The model under review builds one solid part; all positions refer to its coordinate system, in mm. A direction names the side the tool comes from. Round coordinates to 2 decimals unless told otherwise and drop trailing zeros. Loops run counter-clockwise (first coordinate to the right, second up) from the corner with the lowest first, then second, coordinate; pieces in that order, holes last. Notation, with made-up numbers: M 63.5,83 L 114.5,83 A22 ccw 114.5,106 Z; hole C -3,-22.75 d2. An arc over 180 degrees is marked long. Use a Markdown table: item, result. Add a question column.
```python
from build123d import *

# Parameters (mm, degrees)
SALIENTE_EXTRUIR1_DEPTH  = 22
CROQUIS3_R               = 2.5
CROQUIS3_R_2             = 4.5
CORTAR_EXTRUIR2_DEPTH    = 1.5
CROQUIS4_R               = 2.5
CORTAR_EXTRUIR3_DEPTH    = 18
CROQUIS5_R               = 4.05861195
CORTAR_EXTRUIR4_DEPTH    = 1.5
CROQUIS6_R               = 2.5
CORTAR_EXTRUIR5_DEPTH    = 15
SALIENTE_EXTRUIR2_DEPTH  = 19
CROQUIS8_R               = 3
CORTAR_EXTRUIR7_DEPTH    = 19
CROQUIS9_R               = 4
CORTAR_EXTRUIR10_DEPTH   = 0.5
CORTAR_EXTRUIR10_DRAFT   = -80
CROQUIS10_R              = 4
CORTAR_EXTRUIR11_DEPTH   = 0.5
CORTAR_EXTRUIR11_DRAFT   = -80
SALIENTE_EXTRUIR3_DEPTH  = 135.5
CROQUIS12_R              = 10
CORTAR_EXTRUIR12_DEPTH   = 100
CROQUIS15_R              = 18.75
SALIENTE_EXTRUIR10_DEPTH = 80
CROQUIS16_R              = 4
CORTAR_EXTRUIR13_DEPTH   = 151.762230018


with BuildPart() as part:
    # Croquis2 → Saliente-Extruir1 (new body)
    with BuildSketch(Plane(origin=(0, 0, 0), x_dir=(1, 0, 0), z_dir=(0, 1, 0))):
        with BuildLine():
            Line((-17.878262929, 49.088471905), (-10.775937662, 54.088471905))
            ThreePointArc((-10.775937662, 54.088471905), (-9.407250911, 54.766673868), (-7.897674733, 55))
            Line((-7.897674733, 55), (7.897674733, 55))
            ThreePointArc((7.897674733, 55), (9.407250911, 54.766673868), (10.775937662, 54.088471905))
            Line((10.775937662, 54.088471905), (17.878262929, 49.088471905))
            ThreePointArc((17.878262929, 49.088471905), (19.437978968, 47.303115863), (20, 45))
            Line((20, 45), (20, 0))
            ThreePointArc((20, 0), (0, -20), (-20, 0))
            Line((-20, 0), (-20, 45))
            ThreePointArc((-20, 45), (-19.437978968, 47.303115863), (-17.878262929, 49.088471905))
        make_face()
    extrude(amount=SALIENTE_EXTRUIR1_DEPTH)

    # Croquis3 → Cortar-Extruir2 (cut)
    with BuildSketch(Plane(origin=(0, 22, 0), x_dir=(1, 0, 0), z_dir=(0, 1, 0))):
        with Locations(Location((-15, 45, 0), (0, 0, 270))):
            Circle(CROQUIS3_R)
        with Locations(Location((15, 45, 0), (0, 0, 270))):
            Circle(CROQUIS3_R)
        with Locations((-16.5, 36)):
            Circle(CROQUIS3_R_2)
        with Locations((16.5, 36)):
            Circle(CROQUIS3_R_2)
    extrude(amount=-CORTAR_EXTRUIR2_DEPTH, mode=Mode.SUBTRACT)

    # Croquis4 → Cortar-Extruir3 (cut)
    with BuildSketch(Plane(origin=(0, 22, 0), x_dir=(1, 0, 0), z_dir=(0, 1, 0))):
        with Locations(Location((-15, 45, 0), (0, 0, 270))):
            Circle(CROQUIS4_R)
        with Locations(Location((15, 45, 0), (0, 0, 270))):
            Circle(CROQUIS4_R)
    extrude(amount=-CORTAR_EXTRUIR3_DEPTH, mode=Mode.SUBTRACT)

    # Croquis5 → Cortar-Extruir4 (cut)
    with BuildSketch(Plane(origin=(0, 22, 0), x_dir=(1, 0, 0), z_dir=(0, 1, 0))):
        with Locations((0.022007055, -18)):
            Circle(CROQUIS5_R)
    extrude(amount=-CORTAR_EXTRUIR4_DEPTH, mode=Mode.SUBTRACT)

    # Croquis6 → Cortar-Extruir5 (cut)
    with BuildSketch(Plane(origin=(0, 20.5, 0), x_dir=(1, 0, 0), z_dir=(0, 1, 0))):
        with Locations(Location((0.024452265, -16.999985052, 0), (0, 0, 270))):
            Circle(CROQUIS6_R)
    extrude(amount=-CORTAR_EXTRUIR5_DEPTH, mode=Mode.SUBTRACT)

    # Croquis7 → Saliente-Extruir2 (add)
    with BuildSketch(Plane(origin=(0, 20.5, 0), x_dir=(1, 0, 0), z_dir=(0, 1, 0))):
        with BuildLine():
            Line((7, 25), (-7, 25))
            ThreePointArc((-7, 25), (-8.414213562, 25.585786438), (-9, 27))
            Line((-9, 27), (-9, 41))
            ThreePointArc((-9, 41), (-8.414213562, 42.414213562), (-7, 43))
            Line((-7, 43), (7, 43))
            ThreePointArc((7, 43), (8.414213562, 42.414213562), (9, 41))
            Line((9, 41), (9, 27))
            ThreePointArc((9, 27), (8.414213562, 25.585786438), (7, 25))
        make_face()
    extrude(amount=SALIENTE_EXTRUIR2_DEPTH)

    # Croquis8 → Cortar-Extruir7 (cut)
    with BuildSketch(Plane.ZY.offset(9)):
        with Locations((-34, 30.75)):
            Circle(CROQUIS8_R)
    extrude(amount=-CORTAR_EXTRUIR7_DEPTH, mode=Mode.SUBTRACT)


with BuildPart() as cortar_extruir10_tool:
    # Croquis9 → Cortar-Extruir10 (with draft: the straight prism first)
    with BuildSketch(Plane.ZY.offset(9)):
        with Locations((-34, 30.75)):
            Circle(CROQUIS9_R)
    extrude(amount=-CORTAR_EXTRUIR10_DEPTH)
    # Cortar-Extruir10: the draft: its side faces are tilted about the plane it starts from
    cortar_extruir10_sides = [cortar_extruir10_tool.faces().sort_by_distance(p)[0] for p in [
        (-8.75, 30.75, -38),
    ]]
    draft(cortar_extruir10_sides, Plane.ZY.offset(9), CORTAR_EXTRUIR10_DRAFT)


with BuildPart() as part_1:
    add(part.part)

    # Cortar-Extruir10: cut by cortar_extruir10_tool
    add(cortar_extruir10_tool.part, mode=Mode.SUBTRACT)


with BuildPart() as cortar_extruir11_tool:
    # Croquis10 → Cortar-Extruir11 (with draft: the straight prism first)
    with BuildSketch(Plane(origin=(9, 0, 0), x_dir=(0, 0, -1), z_dir=(1, 0, 0))):
        with Locations((34, 30.75)):
            Circle(CROQUIS10_R)
    extrude(amount=-CORTAR_EXTRUIR11_DEPTH)
    # Cortar-Extruir11: the draft: its side faces are tilted about the plane it starts from
    cortar_extruir11_sides = [cortar_extruir11_tool.faces().sort_by_distance(p)[0] for p in [
        (8.75, 30.75, -30),
    ]]
    draft(cortar_extruir11_sides, Plane(origin=(9, 0, 0), x_dir=(0, 0, -1), z_dir=(1, 0, 0)), CORTAR_EXTRUIR11_DRAFT)


with BuildPart() as part_2:
    add(part_1.part)

    # Cortar-Extruir11: cut by cortar_extruir11_tool
    add(cortar_extruir11_tool.part, mode=Mode.SUBTRACT)

    # Croquis11 → Saliente-Extruir3 (add)
    with BuildSketch(Plane.XZ):
        with BuildLine():
            Line((-10, -55), (-14.509357639, -37.805067791))
            ThreePointArc((-14.509357639, -37.805067791), (0, -19), (14.509357639, -37.805067791))
            Line((14.509357639, -37.805067791), (10, -55))
            Line((10, -55), (-10, -55))
        make_face()
    extrude(amount=SALIENTE_EXTRUIR3_DEPTH)

    # Croquis12 → Cortar-Extruir12 (cut)
    with BuildSketch(Plane.XZ.offset(135.5)):
        with Locations(Location((0, -34, 0), (0, 0, 270))):
            Circle(CROQUIS12_R)
    extrude(amount=-CORTAR_EXTRUIR12_DEPTH, mode=Mode.SUBTRACT)

    # Croquis15 → Saliente-Extruir10 (add)
    with BuildSketch(Plane.XZ):
        with Locations(Location((0, 0, 0), (0, 0, 90))):
            Circle(CROQUIS15_R)
    extrude(amount=SALIENTE_EXTRUIR10_DEPTH)

    # Croquis16 → Cortar-Extruir13 (cut, through all)
    with BuildSketch(Plane(origin=(0, 0, -43), x_dir=(-1, 0, 0), z_dir=(0, 0, -1))):
        with Locations((0, 30.75)):
            Circle(CROQUIS16_R)
    extrude(amount=-CORTAR_EXTRUIR13_DEPTH, mode=Mode.SUBTRACT)


solid = part_2.part
```
(1) Consider section A-A, the plane y = -60. Give the boundary of the cut face in (x, z).
(2) Consider section B-B, the plane y = 30.75. Give the boundary of the cut face in (x, z), then the cut area to 3 significant figures.
(3) For faces 1 (the face through (14.04, 13.13, -42.69)), 2 (the face through (3, -86.2, -43.54)), 3 (the face through (-12.223, -66.802, -46.523)), 4 (the face through (-2, 27, -43)), list the 3-axis set-ups (+Z, -Z, +X, -X, +Y, -Y) from which the entire face can be reached by the end or side of a thin tool; tool diameter is ignored.
(4) Draft analysis for pull direction X (two halves, no side actions). For faces 5 (the face through (0, -35.5, -34)), 6 (the face through (9, 27, -36)), 7 (the face through (-14.38, 10.85, -51.55)), state which applies: released by +X, released by -X, zero draft, split by the parting line, or undercut.
(5) Insertion check: pin 1 Ø5.5 at (x, z) = (14.5, -44) entering from +Y; pin 2 Ø12 at (y, z) = (-78.5, 7.5) entering from -X; pin 3 Ø1 at (y, z) = (-46, 7) entering from -X. Each pin has a flat end and moves straight along its axis. Give the tip position at first contact, or say it passes through.
(6) To check wall thickness, follow probe 1 along X at (y, z) = (13.5, -47); probe 2 along Z at (x, y) = (3, -54); probe 3 along X at (y, z) = (-74, -34). State the ranges of each line that lie inside material, in increasing order.
(7) Consider section D-D, the plane z = -9.5. Give the boundary of the cut face in (x, y), then the cut area to 3 significant figures.
(8) Consider section C-C, the plane y = -2.5. Give the boundary of the cut face in (x, z), then the cut area to 3 significant figures.
Found:
| question | item | result |
|---|---|---|
| 1 | outline | C 0,0 d37.5; M -14.51,-37.81 L -10,-55 L 10,-55 L 14.51,-37.81 A15 ccw long Z; hole C 0,-34 d20 |
| 2 | outline | M -9,-41 A2 ccw -7,-43 L -4,-43 L -4,-37 L -8.82,-37 L -9,-38 Z; M -9,-30 L -8.82,-31 L -4,-31 L -4,-25 L -7,-25 A2 ccw -9,-27 Z; M 4,-43 L 7,-43 A2 ccw 9,-41 L 9,-38 L 8.82,-37 L 4,-37 Z; M 4,-31 L 8.82,-31 L 9,-30 L 9,-27 A2 ccw 7,-25 L 4,-25 Z |
| 2 | area | 116 mm^2 |
| 3 | face 1 | +Y |
| 3 | face 2 | -Y |
| 3 | face 3 | -Z, -X, -Y |
| 3 | face 4 | -Z, +X, -X, +Y |
| 4 | face 5 | undercut |
| 4 | face 6 | released by +X |
| 4 | face 7 | released by -X |
| 5 | pin 1 | stops at y = 22 |
| 5 | pin 2 | stops at x = -18.69 |
| 5 | pin 3 | stops at x = -17.59 |
| 6 | probe 1 | x = -19.58 to -16.5, -13.5 to 13.5, 16.5 to 19.58 |
| 6 | probe 2 | z = -55 to -43.54, -24.46 to -19.3, -18.51 to 18.51 |
| 6 | probe 3 | x = -15 to -10, 10 to 15 |
| 7 | outline | M -20,0 L -16.17,0 L -16.17,-80 L 16.17,-80 L 16.17,0 L 20,0 L 20,22 L -20,22 Z |
| 7 | area | 3,470 mm^2 |
| 8 | outline | C 0,0 d37.5; M -14.51,-37.81 L -10,-55 L 10,-55 L 14.51,-37.81 A15 ccw long Z |
| 8 | area | 1,990 mm^2 |
